from build123d import *

# Parameters (mm, degrees)
ESQUISSE3_R                  = 1.5
ENL_V_MAT_EXTRU_1_DEPTH      = 5
R_P_TITION_CIRCULAIRE1_COUNT = 4


with BuildPart() as part:
    # Esquisse1 → Révolution1 (revolve)
    with BuildSketch(Plane(origin=(0, 0, 0), x_dir=(0, 0, -1), z_dir=(1, 0, 0))):
        Polygon((-6, 15.5), (6, 15.5), (6, 13.5), (-4, 13.5), (-4, 9), (-6, 9), align=None)
    revolve(axis=Axis((0, 0, 6), (0, 0, -1)))

    # Esquisse3 → Enlèv. mat.-Extru.1 (cut)
    with BuildSketch(Plane(origin=(0, 15.5, 0), x_dir=(1, 0, 0), z_dir=(0, 1, 0))):
        Circle(ESQUISSE3_R)
    enl_v_mat_extru_1 = extrude(amount=-ENL_V_MAT_EXTRU_1_DEPTH, mode=Mode.SUBTRACT)

    # Répétition circulaire1: Enlèv. mat.-Extru.1 ×4 about axis
    r_p_tition_circulaire1_axis = Axis((0, 0, 6), (0, 0, 1))
    for i in range(1, R_P_TITION_CIRCULAIRE1_COUNT):
        add(enl_v_mat_extru_1.rotate(r_p_tition_circulaire1_axis, i * 360 / R_P_TITION_CIRCULAIRE1_COUNT), mode=Mode.SUBTRACT)


solid = part.part
Geometry check sheet. Reference: the model listing, model coordinates, mm. A direction names the side the tool comes from. Round coordinates to 2 decimals unless told otherwise and drop trailing zeros. Order: outer loops, then holes, each group sorted by start corner. A loop starts at its lowest first (then second) coordinate and runs counter-clockwise, first axis right, second up. Notation, with made-up numbers: M 64,50.5 L 84,50.5 A19 cw 84,59.5 Z; hole C 88,21.25 d1. An arc over 180 degrees is marked long. Answer in a Markdown table with one row per item. Add a question column.
Item 1: Material ranges on L1, parallel to Z at x = -14.8, y = 0; L2, parallel to X at y = 0, z = 5.2; L3, parallel to Z at x = 11.5, y = 0, recorded low to high. Write a range as [from, to].
Item 2: Sectioned sample at B-B, the plane z = 0. Enter the section's corners in (x, y).
Item 3: Sectioned sample at A-A, the plane x = 0. Enter the section's corners in (y, z), plus the area to 3 significant figures.
Item 4: Set-up check for faces 1 (the face through (8.923, -1.172, 5.014)), 2 (the face through (-5.17, 12.47, -0.93)): record each of +Z, -Z, +X, -X, +Y, -Y from which the full face is reachable in a straight line by a thin tool's end or side.
Item 5: Sectioned sample at D-D, the plane x = -7. Enter the section's corners in (y, z), plus the area to 3 significant figures.
Item 6: Depth check by flat-ended pin: pin 1 Ø2 at (y, z) = (-3, 1) entering from +X; pin 2 Ø3 at (x, z) = (6, -3) entering from +Y; pin 3 Ø5 at (x, z) = (-9, -0.5) entering from -Y. Enter the tip coordinate at first touch or a pass-through.
Item 7: Draft check along X on faces 3 (the face through (4.656, 14.784, -0.084)), 4 (the face through (13, -5, -6)), 5 (the face through (-1.5, 14.47, -0.07)). Enter one of: released by +X, released by -X, zero draft, split by the parting line, or undercut.
Filled in:
| question | item | result |
|---|---|---|
| 1 | L1 | z = [-6, -1.5], [1.5, 6] |
| 1 | L2 | x = [-15.5, -9], [9, 15.5] |
| 1 | L3 | z = [4, 6] |
| 2 | outline | M -15.43,-1.5 A15.5 ccw -1.5,-15.43 L -1.5,-13.42 A13.5 cw -13.42,-1.5 Z; M -15.43,1.5 L -13.42,1.5 A13.5 cw -1.5,13.42 L -1.5,15.43 A15.5 ccw Z; M 1.5,-15.43 A15.5 ccw 15.43,-1.5 L 13.42,-1.5 A13.5 cw 1.5,-13.42 Z; M 1.5,13.42 A13.5 cw 13.42,1.5 L 15.43,1.5 A15.5 ccw 1.5,15.43 Z |
| 3 | outline | M -15.5,-6 L -13.5,-6 L -13.5,-1.5 L -15.5,-1.5 Z; M -15.5,1.5 L -13.5,1.5 L -13.5,4 L -9,4 L -9,6 L -15.5,6 Z; M 9,4 L 13.5,4 L 13.5,1.5 L 15.5,1.5 L 15.5,6 L 9,6 Z; M 13.5,-6 L 15.5,-6 L 15.5,-1.5 L 13.5,-1.5 Z |
| 3 | area | 54.0 mm² |
| 4 | face 1 | +Z, -Z |
| 4 | face 2 | -Z |
| 5 | outline | M -13.83,-6 L -11.54,-6 L -11.54,4 L -5.66,4 L -5.66,6 L -13.83,6 Z; M 5.66,4 L 11.54,4 L 11.54,-6 L 13.83,-6 L 13.83,6 L 5.66,6 Z |
| 5 | area | 78.4 mm² |
| 6 | pin 1 | stops at x = 15.37 |
| 6 | pin 2 | stops at y = 14.83 |
| 6 | pin 3 | stops at y = -14.07 |
| 7 | face 3 | split by the parting line |
| 7 | face 4 | zero draft |
| 7 | face 5 | undercut |
